```python
from build123d import *

# Parameters (mm, degrees)
SKETCH1_R           = 1.6
BOSS_EXTRUDE1_DEPTH = 8
SKETCH2_W           = 8
SKETCH2_H           = 90
BOSS_EXTRUDE2_DEPTH = 60
FILLET1_R           = 10
FILLET2_R           = 10
SKETCH3_R           = 4.4
CUT_EXTRUDE1_DEPTH  = 8
FILLET3_R           = 10
FILLET4_R           = 10


with BuildPart() as part:
    # Sketch1 → Boss-Extrude1 (new body)
    with BuildSketch(Plane(origin=(0, 0, 0), x_dir=(1, 0, 0), z_dir=(0, 1, 0))):
        with BuildLine():
            Line((-25.5, 48), (-24.5, 48))
            ThreePointArc((-24.5, 48), (-17.428932188, 50.928932188), (-14.5, 58))
            Line((-14.5, 58), (-14.5, 128))
            ThreePointArc((-14.5, 128), (-11.571067812, 135.071067812), (-4.5, 138))
            Line((-4.5, 138), (35.5, 138))
            Line((35.5, 138), (35.5, 48))
            Line((35.5, 48), (35.5, -38))
            ThreePointArc((35.5, -38), (32.571067812, -45.071067812), (25.5, -48))
            Line((25.5, -48), (-25.5, -48))
            ThreePointArc((-25.5, -48), (-32.571067812, -45.071067812), (-35.5, -38))
            Line((-35.5, -38), (-35.5, 38))
            ThreePointArc((-35.5, 38), (-32.571067812, 45.071067812), (-25.5, 48))
        make_face()
        with Locations((-22.5, 13)):
            Circle(SKETCH1_R, mode=Mode.SUBTRACT)
        with Locations((22.5, 13)):
            Circle(SKETCH1_R, mode=Mode.SUBTRACT)
    extrude(amount=BOSS_EXTRUDE1_DEPTH)

    # Sketch2 → Boss-Extrude2 (add)
    with BuildSketch(Plane.XZ):
        with Locations((31.5, -93)):
            Rectangle(SKETCH2_W, SKETCH2_H)
    extrude(amount=BOSS_EXTRUDE2_DEPTH)

    # Fillet1
    fillet1_edges = [part.edges().sort_by_distance(p)[0] for p in [
        (31.5, -60, -138),
    ]]
    fillet(fillet1_edges, radius=FILLET1_R)

    # Fillet2
    fillet2_edges = [part.edges().sort_by_distance(p)[0] for p in [
        (31.5, -60, -48),
    ]]
    fillet(fillet2_edges, radius=FILLET2_R)

    # Sketch3 → Cut-Extrude1 (cut)
    with BuildSketch(Plane(origin=(35.5, 0, 0), x_dir=(0, 0, -1), z_dir=(1, 0, 0))):
        with Locations((70.5, -25)):
            Circle(SKETCH3_R)
        with Locations((115.5, -25)):
            Circle(SKETCH3_R)
    extrude(amount=-CUT_EXTRUDE1_DEPTH, mode=Mode.SUBTRACT)

    # Fillet3
    fillet3_edges = [part.edges().sort_by_distance(p)[0] for p in [
        (27.5, 0, -93),
    ]]
    fillet(fillet3_edges, radius=FILLET3_R)

    # Fillet4
    fillet4_edges = [part.edges().sort_by_distance(p)[0] for p in [
        (22.5, 0, -48),
    ]]
    fillet(fillet4_edges, radius=FILLET4_R)


solid = part.part
```
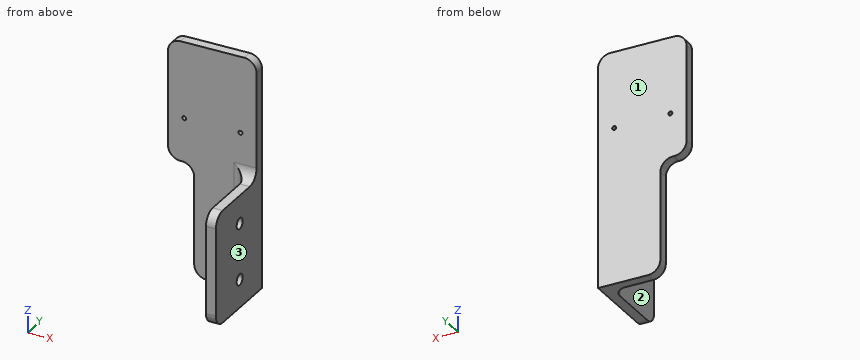
Verification items for the finished model (mm, model axes). Face numbers are marked on the shaded views. Coordinates: 2 decimals unless noted, no trailing zeros. Loops run counter-clockwise (first coordinate to the right, second up) from the corner with the lowest first, then second, coordinate; pieces in that order, holes last. Notation, with made-up numbers: (-31, 85) -> (25, 85) arc R19 ccw to (25, 100) -> close; hole circle Ø9 at (-5.5, 73.25). An arc over 180 degrees is marked (long way). Answer in a Markdown table with one row per item.
1) Depth check by flat-ended pin: P1, Ø9, axis at x = 32.5, y = -32, coming from the +Z side; P2, Ø6.5, axis at y = 6, z = -105, coming from the -X side; P3, Ø10, axis at y = -25, z = -115.5, coming from the +X side; P4, Ø1.5, axis at x = -14, z = -30.5, coming from the -Y side. Enter the tip coordinate at first touch or a pass-through.
The answers:
| item | result |
|---|---|
| P1 | stops at z = -48 |
| P2 | stops at x = -14.5 |
| P3 | stops at x = 35.5 |
| P4 | stops at y = 0 |
2) Section check B-B (z = -115.5). Record the cut outline in (x, y), and give its area (3 significant figures).
The answers:
| item | result |
|---|---|
| outline | (-14.5, 0) -> (17.5, 0) arc R10 cw to (27.5, -10) -> (27.5, -20.6) -> (35.5, -20.6) -> (35.5, 8) -> (-14.5, 8) -> close; (27.5, -60) -> (35.5, -60) -> (35.5, -29.4) -> (27.5, -29.4) -> close |
| area | 831 mm2 |
3) Section check C-C (y = 2.5). Record the cut outline in (x, z), and give its area (3 significant figures).
The answers:
| item | result |
|---|---|
| outline | (-35.5, -38) arc R10 ccw to (-25.5, -48) -> (-24.5, -48) arc R10 cw to (-14.5, -58) -> (-14.5, -128) arc R10 ccw to (-4.5, -138) -> (35.5, -138) -> (35.5, 38) arc R10 ccw to (25.5, 48) -> (-25.5, 48) arc R10 ccw to (-35.5, 38) -> close; hole circle Ø3.2 at (-22.5, -13); hole circle Ø3.2 at (22.5, -13) |
| area | 11,200 mm2 |
4) Section check D-D (z = -51.5). Record the cut outline in (x, y).
The answers:
| item | result |
|---|---|
| outline | (-16.9, 0) -> (17.5, 0) arc R10 cw to (27.5, -10) -> (27.5, -57.6) -> (35.5, -57.6) -> (35.5, 8) -> (-16.9, 8) -> close |
5) Draft check along X on the marked faces 1, 2 and 3. Enter one of: released by +X, released by -X, zero draft, split by the parting line, or undercut.
The answers:
| item | result |
|---|---|
| face 1 | zero draft |
| face 2 | released by -X |
| face 3 | released by +X |
6) Scan lines: line 1 along X through (y, z) = (6, -13); line 2 along Z through (x, y) = (22.5, 1.5); line 3 along X through (y, z) = (-37, -74.5). Record each from-to range of solid material in increasing order. Write a range as from..to.
The answers:
| item | result |
|---|---|
| line 1 | x = -35.5..-24.1, -20.9..20.9, 24.1..35.5 |
| line 2 | z = -138..-14.6, -11.4..48 |
| line 3 | x = 27.5..35.5 |
7) Section check A-A (y = -25). Record the cut outline in (x, z), and give its area (3 significant figures).
The answers:
| item | result |
|---|---|
| outline | (27.5, -138) -> (35.5, -138) -> (35.5, -119.9) -> (27.5, -119.9) -> close; (27.5, -111.1) -> (35.5, -111.1) -> (35.5, -74.9) -> (27.5, -74.9) -> close; (27.5, -66.1) -> (35.5, -66.1) -> (35.5, -48) -> (27.5, -48) -> close |
| area | 579 mm2 |
